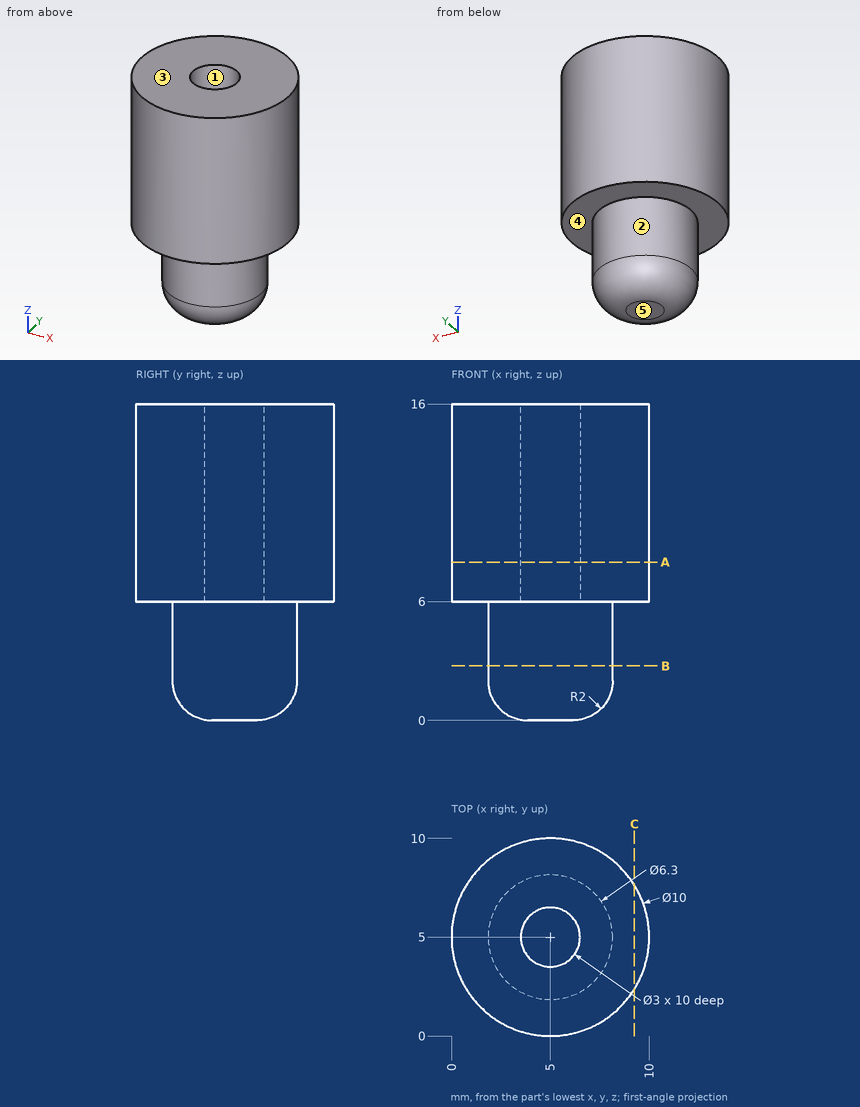
Here's the drawing with two shaded views (mm, measured from the low corner). I have some questions. A direction names the side the tool comes from. Give positions to 0.01 mm unless a question says otherwise; leave off trailing zeros. Order: outer loops, then holes, each group sorted by start corner. A loop starts at its lowest first (then second) coordinate and runs counter-clockwise, first axis right, second up.
Q1. I'm going to push flat-ended pins straight in: P1, Ø1, axis at y = 8, z = 10, coming from the +X side; P2, Ø1.5, axis at x = 4.5, y = 4.5, coming from the +Z side; P3, Ø2, axis at x = 1.5, z = 3.5, coming from the +Y side. Where does each tip first touch, or does it pass through?
Q2. For the marked faces 4 and 5, which set-ups out of +Z, -Z, +X, -X, +Y, -Y let a thin tool reach every point of the face, with its end or its side?
Q3. If I drill on line 1 along Y through (x, z) = (5, 11.5); line 2 along Z through (x, y) = (2, 1.5); line 3 along Z through (x, y) = (5.5, 5), over which ranges is the centre line in solid material (lowest first)?
Q4. Suppose I cut it at A-A, the plane z = 8. Write out the boundary of the cut face in (x, y).
Q5. We'd pull the mould along X, two halves only. Please class the marked faces 1, 2 and 3: +X half, -X half, draft (parallel to the pull), parting line (faces both ways), or undercut.
Q6. Suppose I cut it at B-B, the plane z = 2.75. Write out the boundary of the cut face in (x, y), and give its area (3 significant figures).
Q7. Suppose I cut it at C-C, the plane x = 9.25. Write out the boundary of the cut face in (y, z), and give its area (3 significant figures).
Solution:
1. P1: stops at x = 9.33
1. P2: stops at z = 6
1. P3: stops at y = 6.92
2. face 4: -Z
2. face 5: -Z, +X, -X, +Y, -Y
3. line 1: y = 0 to 3.5, 6.5 to 10
3. line 2: z = 6 to 16
3. line 3: z = 0 to 6
4. outline: circle Ø10 at (5, 5); hole circle Ø3 at (5, 5)
5. face 1: undercut
5. face 2: parting line
5. face 3: draft
6. outline: circle Ø6.3 at (5, 5)
6. area: 31.2 mm2
7. outline: (2.37, 6) - (7.63, 6) - (7.63, 16) - (2.37, 16) - close
7. area: 52.7 mm2
